Design review of the part built by this model. Coordinates are the model's own, in mm. Face numbers are marked on the shaded views. A direction names the side the tool comes from. Coordinates: 2 decimals unless noted, no trailing zeros. Order: outer loops, then holes, each group sorted by start corner. A loop starts at its lowest first (then second) coordinate and runs counter-clockwise, first axis right, second up. Notation, with made-up numbers: M 30,41.5 L 60,41.5 A30 cw 60,75.5 Z; hole C 11,25.25 d2. An arc over 180 degrees is marked long. Use CSV: the item, a comma, the result in double quotes.
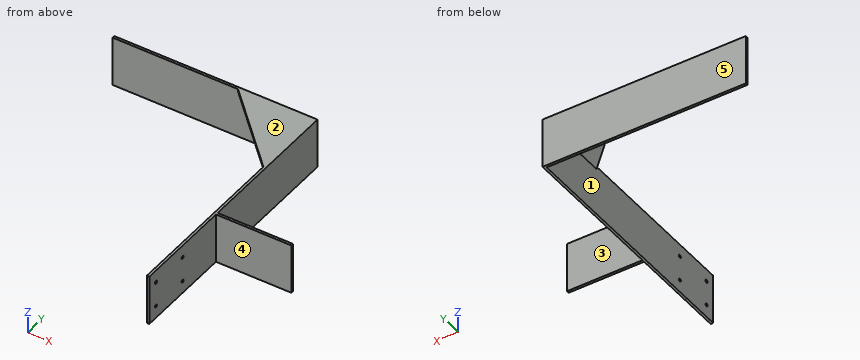
```python
from build123d import *

# Parameters (mm, degrees)
EXTRUDE_THIN1_DEPTH   = 100
F_6_0MM_DOWEL_HOLE1_D = 6
SKETCH8_W             = 100
SKETCH8_H             = 5
BOSS_EXTRUDE3_DEPTH   = 150
BOSS_EXTRUDE4_DEPTH   = 5


with BuildPart() as part:
    # Sketch1 → Extrude-Thin1 (new body)
    with BuildSketch(Plane.XY):
        Polygon((0, 0), (0, 500), (-400, 500), (-400, 505), (5, 505), (5, 0), align=None)
    extrude(amount=EXTRUDE_THIN1_DEPTH)

    # Ø6.0mm Dowel Hole1 (through all)
    with Locations(Plane(origin=(5, 0, 0), x_dir=(0, 0, -1), z_dir=(1, 0, 0))):
        with Locations((-25, 100), (-75, 100), (-75, 20), (-25, 20)):
            Hole(F_6_0MM_DOWEL_HOLE1_D / 2)

    # Sketch8 → Boss-Extrude3 (add)
    with BuildSketch(Plane(origin=(5, 0, 0), x_dir=(0, 0, -1), z_dir=(1, 0, 0))):
        with Locations((-50, 202.5)):
            Rectangle(SKETCH8_W, SKETCH8_H)
    extrude(amount=BOSS_EXTRUDE3_DEPTH)

    # Sketch9 → Boss-Extrude4 (add)
    with BuildSketch(Plane.XY.offset(100)):
        Polygon((-150, 500), (0, 350), (0, 500), align=None)
    extrude(amount=-BOSS_EXTRUDE4_DEPTH)


solid = part.part
```
(1) Clearance check with flat-ended pins moving along their axes: P1, Ø2, axis at x = -262.5, z = 74.5, coming from the -Y side; P2, Ø7, axis at y = 100, z = 25, coming from the -X side; P3, Ø9.5, axis at y = 100, z = 75, coming from the +X side; P4, Ø6, axis at x = -4, y = 181.5, coming from the +Z side. State where each tip first meets the part, or that it passes through.
The answers:
P1,"stops at y = 500"
P2,"stops at x = 0"
P3,"stops at x = 5"
P4,"passes through"
(2) Wall thickness on probe 1 along Y at (x, z) = (2.65, 25); probe 2 along X at (y, z) = (36, 88.5); probe 3 along Y at (x, z) = (-321.5, 28): over which ranges is each line inside the solid? List them lowest first.
The answers:
probe 1,"y = 0 to 17, 23 to 97, 103 to 505"
probe 2,"x = 0 to 5"
probe 3,"y = 500 to 505"
(3) For the marked faces 1, 2, 3, 4 and 5, list the 3-axis set-ups (+Z, -Z, +X, -X, +Y, -Y) from which the entire face can be reached by the end or side of a thin tool; tool diameter is ignored.
The answers:
face 1,"-Z, -X, -Y"
face 2,"+Z, +X, -X, +Y, -Y"
face 3,"+Z, -Z, +X, +Y"
face 4,"+Z, -Z, +X, -Y"
face 5,"+Z, -Z, +X, -X, +Y"
(4) Add section A-A on y = 390.5. State the section outline as (x, z) points, and give its area (4 significant figures).
The answers:
outline,"M -40.5,95 L 0,95 L 0,0 L 5,0 L 5,100 L -40.5,100 Z"
area,"702.5 mm2"
(5) Add section B-B on z = 38. State the section outline as (x, y) points, and give its area (4 significant figures).
The answers:
outline,"M -400,500 L 0,500 L 0,0 L 5,0 L 5,200 L 155,200 L 155,205 L 5,205 L 5,505 L -400,505 Z"
area,"5,275 mm2"
(6) Add section C-C on x = -265. State the section outline as (y, z) points.
The answers:
outline,"M 500,0 L 505,0 L 505,100 L 500,100 Z"
(7) Add section D-D on y = 178. State the section outline as (x, z) points, and give its area (3 significant figures).
The answers:
outline,"M 0,0 L 5,0 L 5,100 L 0,100 Z"
area,"500 mm2"
